from build123d import *

# Parameters (mm, degrees)
BOSS_EXTRUDE1_DEPTH = 6
SKETCH2_R           = 1
SKETCH2_R_2         = 2.25
CUT_EXTRUDE1_DEPTH  = 18.182840277
FILLET1_R           = 4


with BuildPart() as part:
    # Sketch1 → Boss-Extrude1 (new body)
    with BuildSketch(Plane(origin=(0, 0, 0), x_dir=(1, 0, 0), z_dir=(0, 1, 0))):
        Polygon((0, 13), (9.5, 13), (9.5, -8), (6, -8), (6, 0), (0, 0), align=None)
    extrude(amount=BOSS_EXTRUDE1_DEPTH)

    # Sketch2 → Cut-Extrude1 (cut, through all)
    with BuildSketch(Plane(origin=(0, 6, 0), x_dir=(1, 0, 0), z_dir=(0, 1, 0))):
        with Locations((6, -2)):
            Circle(SKETCH2_R)
        with Locations(Location((4.5, 7.5, 0), (0, 0, 270))):
            Circle(SKETCH2_R_2)
        with Locations((6, -6)):
            Circle(SKETCH2_R)
    extrude(amount=-CUT_EXTRUDE1_DEPTH, mode=Mode.SUBTRACT)

    # Fillet1
    fillet1_edges = [part.edges().sort_by_distance(p)[0] for p in [
        (0, 3, -13),
        (9.5, 3, -13),
    ]]
    fillet(fillet1_edges, radius=FILLET1_R)


solid = part.part
Verification items for the finished model (mm, model axes). A direction names the side the tool comes from. Round coordinates to 2 decimals unless told otherwise and drop trailing zeros. Loops run counter-clockwise (first coordinate to the right, second up) from the corner with the lowest first, then second, coordinate; pieces in that order, holes last. Notation, with made-up numbers: (55.25, -22.5) - (78.25, -22.5) arc R21 cw to (78.25, -14.5) - close; hole circle Ø11 at (-9.75, 80). An arc over 180 degrees is marked (long way). Use one line per item in the form item = value.
1. Scan lines: probe 1 along X at (y, z) = (2.4, -7.5); probe 2 along Z at (x, y) = (5, 1.65); probe 3 along Z at (x, y) = (6.5, 2.2). Record each from-to range of solid material in increasing order.
A:
probe_1 = 0 to 2.25, 6.75 to 9.5
probe_2 = -13 to -9.69, -5.31 to 0
probe_3 = -12.87 to -8.53, -6.47 to 1.13, 2.87 to 5.13, 6.87 to 8
2. Access from +Z, -Z, +X, -X, +Y, -Y to the whole of each face (thin tool, end or side, straight path). Record for faces 5 (the flat face through (6, 3, 7.5)), 6 (the flat face through (0, 3, -4)).
A:
face_5 = +Z, -X, +Y, -Y
face_6 = +Z, -Z, -X, +Y, -Y
3. Section check C-C on y = 2.8. Record the cut outline in (x, z), and give its area (3 significant figures).
A:
outline = (0, -9) arc R4 ccw to (4, -13) - (5.5, -13) arc R4 ccw to (9.5, -9) - (9.5, 8) - (6, 8) - (6, 7) arc R1 cw to (6, 5) - (6, 3) arc R1 cw to (6, 1) - (6, 0) - (0, 0) - close; hole circle Ø4.5 at (4.5, -7.5)
area = 126 mm²
4. Section check A-A on x = 4.5. Record the cut outline in (y, z).
A:
outline = (0, -13) - (6, -13) - (6, -9.75) - (0, -9.75) - close; (0, -5.25) - (6, -5.25) - (6, 0) - (0, 0) - close
5. Section check B-B on z = -7.5. Record the cut outline in (x, y), and give its area (3 significant figures).
A:
outline = (0, 0) - (2.25, 0) - (2.25, 6) - (0, 6) - close; (6.75, 0) - (9.5, 0) - (9.5, 6) - (6.75, 6) - close
area = 30.0 mm²
6. Draft check along X on faces 1 (the cylindrical face through (8.297, 3.042, -11.859)), 2 (the cylindrical face through (4.599, 3.042, -9.748)), 3 (the flat face through (3, 3, 0)), 4 (the cylindrical face through (1.203, 3.042, -11.859)). Enter one of: pulls with the +X half, pulls with the -X half, needs draft (parallel to the pull), parting line crosses it, or undercut.
A:
face_1 = pulls with the +X half
face_2 = undercut
face_3 = needs draft
face_4 = pulls with the -X half
7. Gauge pin test, flat end, axial feed: pin 1 Ø0.6 at (y, z) = (4.5, 4.5) entering from -X. Record the tip position at first contact, or that the pin passes through.
A:
pin_1 = 6
8. Section check D-D on z = 6. Record the cut outline in (x, y).
A:
outline = (7, 0) - (9.5, 0) - (9.5, 6) - (7, 6) - close
